Check sheet for the drawn part. Datum: minimum x, y, z corner. Units: mm. Round coordinates to 2 decimals unless told otherwise and drop trailing zeros. Loops run counter-clockwise (first coordinate to the right, second up) from the corner with the lowest first, then second, coordinate; pieces in that order, holes last. Notation, with made-up numbers: (80.25, 65.5) - (115.25, 65.5) arc R19 ccw to (115.25, 80.5) - close; hole circle Ø3 at (33, -27.75). An arc over 180 degrees is marked (long way). Use CSV: the item, a comma, the result in double quotes.
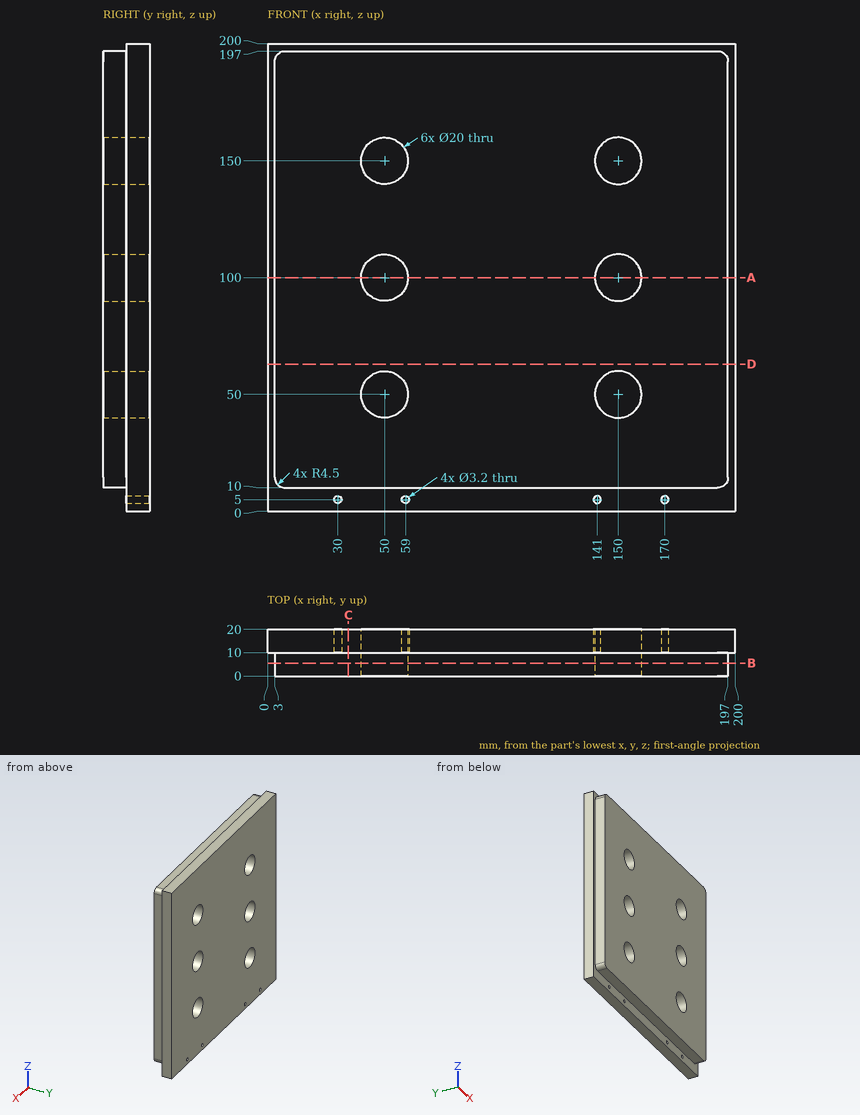
1) Cross-section at D-D, the plane z = 63. Record the cut outline in (x, y).
Returned:
outline,"(0, 10) - (3, 10) - (3, 0) - (197, 0) - (197, 10) - (200, 10) - (200, 20) - (0, 20) - close"
2) Thickness scan on probe 1 along Z at (x, y) = (150, 6.5); probe 2 along X at (y, z) = (12.5, 150); probe 3 along X at (y, z) = (7.75, 150). Record the ranges inside material, lowest first. Write a range as [from, to].
Returned:
probe 1,"z = [10, 40], [60, 90], [110, 140], [160, 197]"
probe 2,"x = [0, 40], [60, 140], [160, 200]"
probe 3,"x = [3, 40], [60, 140], [160, 197]"
3) Gauge pin test, flat ends, axial feed: pin 1 Ø8 at (y, z) = (3, 98) entering from -X; pin 2 Ø12 at (x, y) = (65, 9) entering from -Z. Record the tip position at first contact, or that the pin passes through.
Returned:
pin 1,"stops at x = 3"
pin 2,"stops at z = 0"
4) Cross-section at B-B, the plane y = 5.5. Record the cut outline in (x, z).
Returned:
outline,"(3, 14.5) arc R4.5 ccw to (7.5, 10) - (192.5, 10) arc R4.5 ccw to (197, 14.5) - (197, 192.5) arc R4.5 ccw to (192.5, 197) - (7.5, 197) arc R4.5 ccw to (3, 192.5) - close; hole circle Ø20 at (50, 50); hole circle Ø20 at (50, 100); hole circle Ø20 at (50, 150); hole circle Ø20 at (150, 50); hole circle Ø20 at (150, 100); hole circle Ø20 at (150, 150)"
5) Cross-section at C-C, the plane x = 34.5. Record the cut outline in (y, z).
Returned:
outline,"(0, 10) - (10, 10) - (10, 0) - (20, 0) - (20, 200) - (10, 200) - (10, 197) - (0, 197) - close"
6) Cross-section at A-A, the plane z = 100. Record the cut outline in (x, y).
Returned:
outline,"(0, 10) - (3, 10) - (3, 0) - (40, 0) - (40, 20) - (0, 20) - close; (60, 0) - (140, 0) - (140, 20) - (60, 20) - close; (160, 0) - (197, 0) - (197, 10) - (200, 10) - (200, 20) - (160, 20) - close"
